Input: part model. Units: mm. Frame: model coordinates. A direction names the side the tool comes from. Coordinates: 2 decimals unless noted, no trailing zeros. Order: outer loops, then holes, each group sorted by start corner. A loop starts at its lowest first (then second) coordinate and runs counter-clockwise, first axis right, second up. Notation, with made-up numbers: M -39,15.25 L -13,15.25 A12 ccw -13,20.25 Z; hole C 84.25,-26.5 d9. An arc over 180 degrees is marked long. One line per item, written item: value.
```python
from build123d import *

# Parameters (mm, degrees)
SKETCH1_R           = 3.3274
BOSS_EXTRUDE1_DEPTH = 114.3


with BuildPart() as part:
    # Sketch1 → Boss-Extrude1 (new body, symmetric)
    with BuildSketch(Plane.XY):
        with BuildLine():
            Line((-4.064, 16.539617552), (-4.064, 17.496382454))
            ThreePointArc((-4.064, 17.496382454), (-4.519044044, 18.594955958), (-5.617617547, 19.050000004))
            Line((-5.617617547, 19.050000004), (-15.84748704, 19.050000004))
            ThreePointArc((-15.84748704, 19.050000004), (-18.12017629, 18.120192086), (-19.050000001, 15.847509297))
            Line((-19.050000001, 15.847509297), (-19.050000001, 5.617617549))
            ThreePointArc((-19.050000001, 5.617617549), (-18.594955957, 4.519044045), (-17.496382454, 4.064))
            Line((-17.496382454, 4.064), (-16.539617549, 4.064))
            ThreePointArc((-16.539617549, 4.064), (-15.441044044, 4.519044045), (-14.986, 5.617617549))
            Line((-14.986, 5.617617549), (-14.986, 9.385342517))
            ThreePointArc((-14.986, 9.385342517), (-14.721898184, 10.022940701), (-14.0843, 10.287042517))
            Line((-14.0843, 10.287042517), (-13.516042086, 10.287042517))
            ThreePointArc((-13.516042086, 10.287042517), (-13.170975923, 10.218404479), (-12.878443117, 10.022939917))
            Line((-12.878443117, 10.022939917), (-8.14758008, 5.292065242))
            ThreePointArc((-8.14758008, 5.292065242), (-7.117955877, 3.751120652), (-6.756399998, 1.933453582))
            Line((-6.756399998, 1.933453582), (-6.756399998, -1.933453584))
            ThreePointArc((-6.756399998, -1.933453584), (-7.117955877, -3.751120652), (-8.147580078, -5.292065242))
            Line((-8.147580078, -5.292065242), (-12.878443116, -10.022939917))
            ThreePointArc((-12.878443116, -10.022939917), (-13.170975922, -10.21840448), (-13.516042086, -10.287042518))
            Line((-13.516042086, -10.287042518), (-14.0843, -10.287042518))
            ThreePointArc((-14.0843, -10.287042518), (-14.721898185, -10.022940703), (-14.986, -9.385342518))
            Line((-14.986, -9.385342518), (-14.986, -5.617617549))
            ThreePointArc((-14.986, -5.617617549), (-15.441044044, -4.519044046), (-16.539617547, -4.064))
            Line((-16.539617547, -4.064), (-17.496382452, -4.064))
            ThreePointArc((-17.496382452, -4.064), (-18.594955956, -4.519044044), (-19.050000001, -5.617617547))
            Line((-19.050000001, -5.617617547), (-19.050000001, -15.84751072))
            ThreePointArc((-19.050000001, -15.84751072), (-18.120175718, -18.120192644), (-15.84748687, -19.050000001))
            Line((-15.84748687, -19.050000001), (-5.617617549, -19.050000001))
            ThreePointArc((-5.617617549, -19.050000001), (-4.519044046, -18.594955957), (-4.064, -17.496382454))
            Line((-4.064, -17.496382454), (-4.064, -16.539617549))
            ThreePointArc((-4.064, -16.539617549), (-4.519044045, -15.441044044), (-5.617617549, -14.985999999))
            Line((-5.617617549, -14.985999999), (-9.3853, -14.985999999))
            ThreePointArc((-9.3853, -14.985999999), (-10.022898185, -14.721898184), (-10.287, -14.084299999))
            Line((-10.287, -14.084299999), (-10.287, -13.552357131))
            ThreePointArc((-10.287, -13.552357131), (-10.218362387, -13.207291993), (-10.022898969, -12.914759731))
            Line((-10.022898969, -12.914759731), (-5.252158104, -8.14400713))
            ThreePointArc((-5.252158104, -8.14400713), (-3.715177371, -7.117027388), (-1.902183976, -6.7564))
            Line((-1.902183976, -6.7564), (1.902183976, -6.7564))
            ThreePointArc((1.902183976, -6.7564), (3.715177372, -7.117027388), (5.252158106, -8.144007132))
            Line((5.252158106, -8.144007132), (10.022898969, -12.91475973))
            ThreePointArc((10.022898969, -12.91475973), (10.218362387, -13.207291993), (10.287000001, -13.552357132))
            Line((10.287000001, -13.552357132), (10.287000001, -14.0843))
            ThreePointArc((10.287000001, -14.0843), (10.022898185, -14.721898184), (9.385300001, -14.986))
            Line((9.385300001, -14.986), (5.617617549, -14.986))
            ThreePointArc((5.617617549, -14.986), (4.519044045, -15.441044044), (4.064, -16.539617547))
            Line((4.064, -16.539617547), (4.064, -17.496382452))
            ThreePointArc((4.064, -17.496382452), (4.519044043, -18.594955955), (5.617617546, -19.050000001))
            Line((5.617617546, -19.050000001), (15.847486867, -19.050000001))
            ThreePointArc((15.847486867, -19.050000001), (18.120175716, -18.120192646), (19.05, -15.847510723))
            Line((19.05, -15.847510723), (19.05, -5.617617549))
            ThreePointArc((19.05, -5.617617549), (18.594955955, -4.519044045), (17.496382451, -4.064))
            Line((17.496382451, -4.064), (16.539617548, -4.064))
            ThreePointArc((16.539617548, -4.064), (15.441044044, -4.519044045), (14.985999999, -5.617617549))
            Line((14.985999999, -5.617617549), (14.985999999, -9.385342517))
            ThreePointArc((14.985999999, -9.385342517), (14.721898184, -10.022940701), (14.084299999, -10.287042517))
            Line((14.084299999, -10.287042517), (13.516042085, -10.287042517))
            ThreePointArc((13.516042085, -10.287042517), (13.170975922, -10.218404479), (12.878443117, -10.022939917))
            Line((12.878443117, -10.022939917), (8.147580079, -5.292065242))
            ThreePointArc((8.147580079, -5.292065242), (7.117955877, -3.751120652), (6.756399998, -1.933453583))
            Line((6.756399998, -1.933453583), (6.756399998, 1.933453583))
            ThreePointArc((6.756399998, 1.933453583), (7.117955877, 3.751120652), (8.147580078, 5.292065242))
            Line((8.147580078, 5.292065242), (12.878443116, 10.022939916))
            ThreePointArc((12.878443116, 10.022939916), (13.170975922, 10.218404477), (13.516042084, 10.287042515))
            Line((13.516042084, 10.287042515), (14.084299998, 10.287042515))
            ThreePointArc((14.084299998, 10.287042515), (14.721898183, 10.0229407), (14.985999998, 9.385342515))
            Line((14.985999998, 9.385342515), (14.985999998, 5.617617546))
            ThreePointArc((14.985999998, 5.617617546), (15.441044043, 4.519044042), (16.539617547, 4.063999997))
            Line((16.539617547, 4.063999997), (17.49638245, 4.063999997))
            ThreePointArc((17.49638245, 4.063999997), (18.594955956, 4.519044042), (19.05, 5.617617548))
            Line((19.05, 5.617617548), (19.05, 15.8475093))
            ThreePointArc((19.05, 15.8475093), (18.120176289, 18.120192086), (15.847487041, 19.050000004))
            Line((15.847487041, 19.050000004), (5.617617548, 19.050000004))
            ThreePointArc((5.617617548, 19.050000004), (4.519044044, 18.594955959), (4.063999999, 17.496382454))
            Line((4.063999999, 17.496382454), (4.063999999, 16.539617552))
            ThreePointArc((4.063999999, 16.539617552), (4.519044044, 15.441044047), (5.617617548, 14.986000002))
            Line((5.617617548, 14.986000002), (9.385299999, 14.986000002))
            ThreePointArc((9.385299999, 14.986000002), (10.022898183, 14.721898187), (10.286999999, 14.084300002))
            Line((10.286999999, 14.084300002), (10.286999999, 13.552357134))
            ThreePointArc((10.286999999, 13.552357134), (10.218362386, 13.207291996), (10.022898968, 12.914759734))
            Line((10.022898968, 12.914759734), (5.252158103, 8.144007133))
            ThreePointArc((5.252158103, 8.144007133), (3.71517737, 7.117027391), (1.902183975, 6.756400003))
            Line((1.902183975, 6.756400003), (-1.902183977, 6.756400003))
            ThreePointArc((-1.902183977, 6.756400003), (-3.715177373, 7.117027391), (-5.252158106, 8.144007134))
            Line((-5.252158106, 8.144007134), (-10.022898969, 12.914759733))
            ThreePointArc((-10.022898969, 12.914759733), (-10.218362387, 13.207291995), (-10.287000001, 13.552357134))
            Line((-10.287000001, 13.552357134), (-10.287000001, 14.084300002))
            ThreePointArc((-10.287000001, 14.084300002), (-10.022898186, 14.721898187), (-9.385300001, 14.986000002))
            Line((-9.385300001, 14.986000002), (-5.617617549, 14.986000002))
            ThreePointArc((-5.617617549, 14.986000002), (-4.519044044, 15.441044047), (-4.064, 16.539617552))
        make_face()
        Circle(SKETCH1_R, mode=Mode.SUBTRACT)
    extrude(amount=BOSS_EXTRUDE1_DEPTH, both=True)


solid = part.part
```
(1) Access query for faces 1 (the flat face through (0, -6.756, 2)), 2 (the flat face through (-11, -19.05, 2)), 3 (the flat face through (7, 14.986, 2)). Directions: +Z, -Z, +X, -X, +Y, -Y. A direction counts if a zero-diameter tool reaches every point of the face in a straight line with its end or side. Return the directions, or none.
Data:
face 1: +Z, -Z, -Y
face 2: +Z, -Z, +X, -X, -Y
face 3: +Z, -Z
(2) Draft query along X for faces 4 (the flat face through (-19.05, 11, 2)), 5 (the flat face through (19.05, -11, 2)), 6 (the flat face through (-14.986, 7, 2)). Return one class per face: released by +X, released by -X, zero draft, split by the parting line, or undercut.
Data:
face 4: released by -X
face 5: released by +X
face 6: undercut
(3) First-contact query: pin 1 (8 mm diameter, centred on x = 13, y = -1, fed in from +Z); pin 2 (1.2 mm diameter, centred on y = 1, z = 52, fed in from -X); pin 3 (1.5 mm diameter, centred on y = 3, z = -58.5, fed in from +X); pin 4 (6 mm diameter, centred on x = 1.5, z = -31.5, fed in from +Y). Flat tips, straight axial feed; report the tip coordinate or a pass-through.
Data:
pin 1: passes through
pin 2: stops at x = -6.76
pin 3: stops at x = 7.12
pin 4: stops at y = 18.58
(4) Ray query, line 1 (Y direction, x = 0, z = 68); line 2 (X direction, y = 6.5, z = 56.5); line 3 (X direction, y = 9, z = -87.5). Return the intervals inside material, ascending. Write a range as from..to.
Data:
line 1: y = -6.76..-3.33, 3.33..6.76
line 2: x = -19.05..-14.99, -9.36..9.36, 14.99..19.05
line 3: x = -19.05..-14.99, -11.86..-6.11, 6.11..11.86, 14.99..19.05
(5) Cut plane A-A on x = 0. Output: boundary loops of the cut face in (y, z).
Data:
outline: M -6.76,-114.3 L -3.33,-114.3 L -3.33,114.3 L -6.76,114.3 Z; M 3.33,-114.3 L 6.76,-114.3 L 6.76,114.3 L 3.33,114.3 Z
